Model file for the job. Use its own axes, mm. A direction names the side the tool comes from. Coordinates: 2 decimals unless noted, no trailing zeros. Write each loop counter-clockwise with the first axis right and the second up, starting at its lowest first coordinate (ties: lowest second). Pieces come first, ordered by that corner, then holes. Notation, with made-up numbers: M -20.75,-9 L -3.75,-9 A11 ccw -3.75,2 Z; hole C -3,-28 d8. An arc over 180 degrees is marked long. Put each result on its own line as item: value. Start each with the question number.
Q1. Cut at C-C (z = -2). Write the cut outline in (x, y).
Q2. Drop flat-ended pins along their axis: pin 1 (8 mm diameter, centred on x = -3.5, y = -14.5, fed in from -Z); pin 2 (3 mm diameter, centred on x = 30, y = -12.5, fed in from -Z); pin 3 (10 mm diameter, centred on x = 27, y = 6, fed in from +Z); pin 4 (8 mm diameter, centred on x = 5.5, y = -4.5, fed in from +Z). Give the stop position or say it passes through.
Q3. Cut at B-B (y = 12.5). Write the cut outline in (x, z).
Q4. Cut at D-D (y = -9.5). Write the cut outline in (x, z).
Q5. Cut at A-A (x = 30). Write the cut outline in (y, z), then the cut area to 3 significant figures.
Q6. Which spindle directions (+Z, -Z, +X, -X, +Y, -Y) get a long thin tool onto all of the face, cutting with end or side? Do faces 4 (the flat face through (30, 0, 0)), 5 (the cylindrical face through (-11.92, -0.35, 6.24)). Say none if no direction does.
Q7. Pull direction Y, two halves, no side cores. Call faces 1 (the flat face through (22, 0, -10.668)), 2 (the flat face through (19.1, -25, -0.2)), 3 (the cylindrical face through (28.3, 14.05, -5.26)): pulls with the +Y half, pulls with the -Y half, needs draft (parallel to the pull), parting line crosses it, or undercut.
Q8. Drill centre lines: line 1 along Y through (x, z) = (30, -5.75); line 2 along X through (y, z) = (1, 9.75); line 3 along Z through (x, y) = (34, 4). Where is each one in solid material? Low to high.
```python
from build123d import *

# Parameters (mm, degrees)
F1_DEPTH = 25
F2_R     = 5
F3_R     = 2.3
F4_DEPTH = 10.669


with BuildPart() as f1:
    # F0 (on Front) → F1 (new body, symmetric)
    with BuildSketch(Plane.XZ):
        with BuildLine():
            ThreePointArc((-8.367673, 6.617271), (6.617271, 8.367673), (8.367673, -6.617271))
            ThreePointArc((8.367673, -6.617271), (8.078399, -9.257307), (10.328601, -10.668))
            Line((10.328601, -10.668), (40, -10.668))
            Line((40, -10.668), (40, 0))
            Line((40, 0), (15.668, 0))
            ThreePointArc((15.668, 0), (5.144603, 14.7993), (-12.289529, 9.718729))
            ThreePointArc((-12.289529, 9.718729), (-11.87933, 6.207072), (-8.367673, 6.617271))
        make_face()
    extrude(amount=F1_DEPTH, both=True)

    # F2
    f2_edges = [f1.edges().sort_by_distance(p)[0] for p in [
        (15.668, 0, 0),
        (40, 0, -10.668),
    ]]
    fillet(f2_edges, radius=F2_R)

    # F3 (on Top) → F4 (cut, through all)
    with BuildSketch(Plane.XY):
        with Locations((30, 12.5)):
            Circle(F3_R)
        with Locations((30, -12.5)):
            Circle(F3_R)
    extrude(amount=-F4_DEPTH, mode=Mode.SUBTRACT)


solid = f1.part
```
Computed values:
1. outline: M 10.48,-25 L 40,-25 L 40,25 L 10.48,25 Z; hole C 30,-12.5 d4.6; hole C 30,12.5 d4.6
2. pin 1: z = 7.59
2. pin 2: through
2. pin 3: z = 0
2. pin 4: z = 15.6
3. outline: M -12.29,9.72 A2.5 ccw -8.37,6.62 A10.67 cw 8.37,-6.62 A2.5 ccw 10.33,-10.67 L 27.7,-10.67 L 27.7,0 L 20.05,0 A5 cw 15.2,3.79 A15.67 ccw Z; M 32.3,-10.67 L 35,-10.67 A5 ccw 40,-5.67 L 40,0 L 32.3,0 Z
4. outline: M -12.29,9.72 A2.5 ccw -8.37,6.62 A10.67 cw 8.37,-6.62 A2.5 ccw 10.33,-10.67 L 35,-10.67 A5 ccw 40,-5.67 L 40,0 L 20.05,0 A5 cw 15.2,3.79 A15.67 ccw Z
5. outline: M -25,-10.67 L -14.8,-10.67 L -14.8,0 L -25,0 Z; M -10.2,-10.67 L 10.2,-10.67 L 10.2,0 L -10.2,0 Z; M 14.8,-10.67 L 25,-10.67 L 25,0 L 14.8,0 Z
5. area: 435 mm2
6. face 4: +Z, +X, +Y, -Y
6. face 5: +Y, -Y
7. face 1: needs draft
7. face 2: pulls with the -Y half
7. face 3: undercut
8. line 1: -25 to -14.8, -10.2 to 10.2, 14.8 to 25
8. line 2: -12.26 to -4.33, 4.33 to 12.26
8. line 3: -10.67 to 0
